Answer from the drawing. Dimensions are ordinates in mm from the lowest x, y and z of the part. Give positions to 0.01 mm unless a question says otherwise; leave off trailing zeros. Write each loop counter-clockwise with the first axis right and the second up, starting at its lowest first coordinate (ties: lowest second). Pieces come first, ordered by that corner, then holes. Notation, with made-up numbers: M 32.25,85.25 L 36.25,85.25 A20 cw 36.25,120.25 Z; hole C 54,-24 d10. An arc over 180 degrees is marked long. Put each result on its own line as item: value.
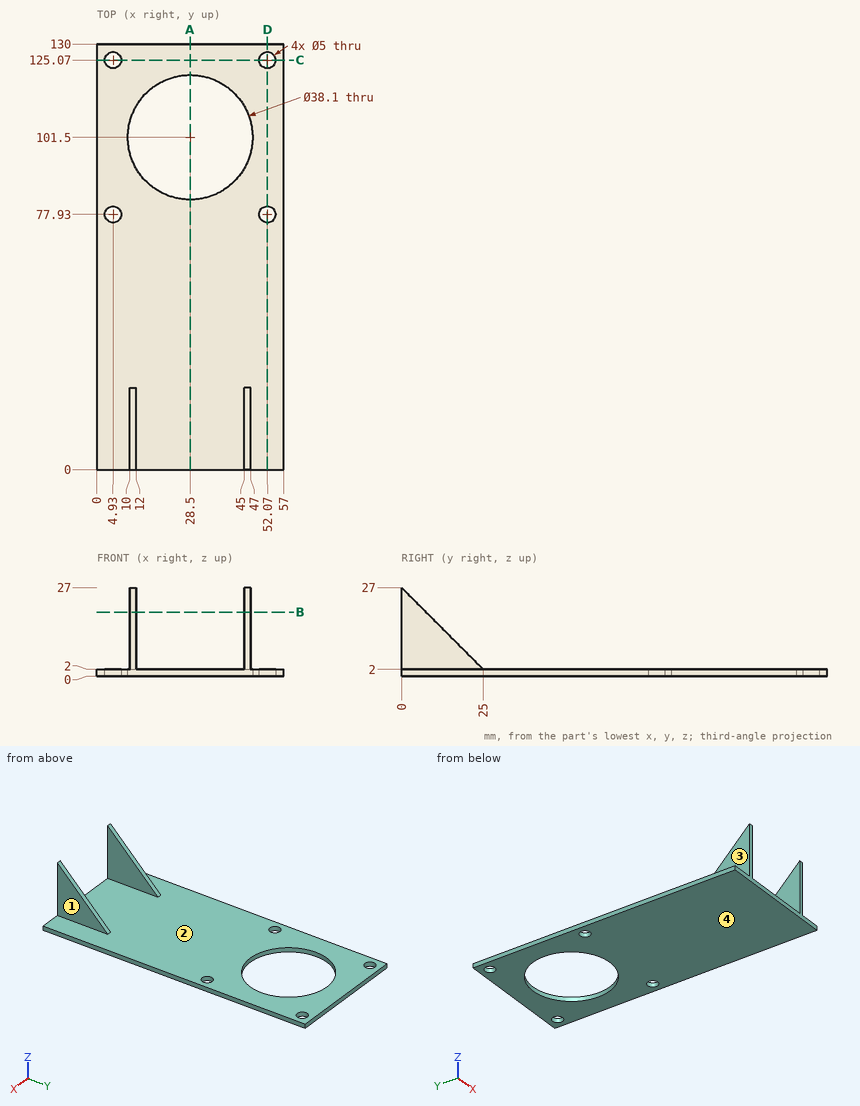
(1) For a pull along X with two mould halves and no side action, classify the marked faces 1, 2, 3 and 4 as +X half, -X half, draft (parallel to the pull), parting line (faces both ways), or undercut.
Result:
face 1: +X half
face 2: undercut
face 3: -X half
face 4: draft
(2) Section B-B on z = 19.5 is taken. Determine the outline of the cut face in (x, y), and give its area (3 significant figures).
Result:
outline: M 10,0 L 12,0 L 12,7.5 L 10,7.5 Z; M 45,0 L 47,0 L 47,7.5 L 45,7.5 Z
area: 30.0 mm²
(3) Section C-C on y = 125.07 is taken. Determine the outline of the cut face in (x, z).
Result:
outline: M 0,0 L 2.43,0 L 2.43,2 L 0,2 Z; M 7.43,0 L 49.57,0 L 49.57,2 L 7.43,2 Z; M 54.57,0 L 57,0 L 57,2 L 54.57,2 Z
(4) Section A-A on x = 28.5 is taken. Determine the outline of the cut face in (y, z), and give its area (3 significant figures).
Result:
outline: M 0,0 L 82.45,0 L 82.45,2 L 0,2 Z; M 120.55,0 L 130,0 L 130,2 L 120.55,2 Z
area: 184 mm²
(5) Given pin 1 Ø6 at (y, z) = (15, 7.5) entering from -X; pin 2 Ø12.5 at (y, z) = (13, 13) entering from +X; pin 3 Ø12 at (x, z) = (45, 19) entering from +Y, each flat-ended and moving along its own axis, determine where each tip first touches the part or whether it passes through.
Result:
pin 1: stops at x = 10
pin 2: stops at x = 47
pin 3: stops at y = 14
(6) Section D-D on x = 52.07 is taken. Determine the outline of the cut face in (y, z).
Result:
outline: M 0,0 L 75.43,0 L 75.43,2 L 0,2 Z; M 80.43,0 L 122.57,0 L 122.57,2 L 80.43,2 Z; M 127.57,0 L 130,0 L 130,2 L 127.57,2 Z
(7) Straight lines are drawn through the part: line 1 along Y through (x, z) = (4.93, 1); line 2 along Z through (x, y) = (41.5, 66.5). For each, find the intervals that lie inside material, in ascending order. Write a range as from..to.
Result:
line 1: y = 0..75.43, 80.43..122.57, 127.57..130
line 2: z = 0..2
